The model under review builds one solid part; all positions refer to its coordinate system, in mm. Round coordinates to 2 decimals unless told otherwise and drop trailing zeros. Loops run counter-clockwise (first coordinate to the right, second up) from the corner with the lowest first, then second, coordinate; pieces in that order, holes last. Notation, with made-up numbers: M 82.25,17 L 123.25,17 A36 cw 123.25,51 Z; hole C -29.5,-22 d10. An arc over 180 degrees is marked long. Answer in a Markdown table with one row per item. Add a question column.
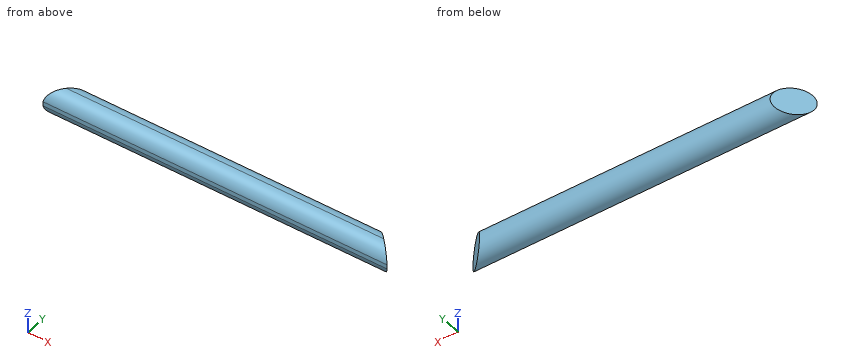
from build123d import *

# Parameters (mm, degrees)
SKETCH2_W               = 1600
SKETCH2_H               = 63.75
CUT_EXTRUDE2_DEPTH      = 1607.337546252
CUT_EXTRUDE2_DEPTH_BACK = 1607.337546252
CUT_EXTRUDE3_DEPTH      = 1607.337546252


with BuildPart() as part:
    # Sketch2 → Revolve1 (revolve)
    with BuildSketch(Plane(origin=(0, 0, 0), x_dir=(1, 0, 0), z_dir=(0, 1, 0))):
        with Locations((800, 31.875)):
            Rectangle(SKETCH2_W, SKETCH2_H)
    revolve(axis=Axis((1600, 0, -63.75), (-1, 0, 0)))

    # Sketch3 → Cut-Extrude2 (cut, two sides: drawn at the far end of the back side and taken through both)
    with BuildSketch(Plane.XY.offset(-CUT_EXTRUDE2_DEPTH_BACK)):
        Polygon((0, 63.75), (125, 63.75), (0, -63.75), align=None)
        Polygon((1600, 63.75), (1600, -63.75), (1475, 63.75), align=None)
    extrude(amount=CUT_EXTRUDE2_DEPTH + CUT_EXTRUDE2_DEPTH_BACK, mode=Mode.SUBTRACT)

    # Sketch5 → Cut-Extrude3 (cut, through all)
    with BuildSketch(Plane(origin=(0, 0, 0), x_dir=(0, 0, -1), z_dir=(1, 0, 0))):
        Polygon((63.75, -63.75), (0, -63.75), (0, -62.96232629), (127.5, -62.96232629), (127.5, -63.75), align=None)
    extrude(amount=CUT_EXTRUDE3_DEPTH, mode=Mode.SUBTRACT)


solid = part.part
1. Take a section at B-B, the plane x = 755.5. State the section outline as (y, z) points.
2. Take a section at C-C, the plane y = 49. State the section outline as (x, z) points, and give its area (3 significant figures).
3. Take a section at A-A, the plane z = -102. State the section outline as (x, y) points, and give its area (3 significant figures).
4. To check wall thickness, follow probe 1 along Z at (x, y) = (1393, 4); probe 2 along Z at (x, y) = (579.5, -1); probe 3 along Y at (x, z) = (494.5, -65). State the ranges of each line that lie inside material, in increasing order.
5. For pin 1 Ø6 at (y, z) = (-17.5, -22) entering from -X; pin 2 Ø2 at (x, y) = (384, -33) entering from +Z; pin 3 Ø1 at (x, y) = (670.5, 31) entering from -Z, all flat-tipped, find the tip position at first contact; note any pin that passes through.
Check sheet entries:
| question | item | result |
|---|---|---|
| 1 | outline | M -62.96,-73.74 A63.75 ccw long -62.96,-53.76 Z |
| 2 | outline | M 110.54,-104.53 L 1489.46,-104.53 L 1489.46,-22.97 L 110.54,-22.97 Z |
| 2 | area | 112,000 mm^2 |
| 3 | outline | M 12.5,-51 L 1587.5,-51 L 1487.5,51 L 112.5,51 Z |
| 3 | area | 150,000 mm^2 |
| 4 | probe 1 | z = -127.37 to -0.13 |
| 4 | probe 2 | z = -127.49 to -0.01 |
| 4 | probe 3 | y = -62.96 to 63.74 |
| 5 | pin 1 | stops at x = 42.4 |
| 5 | pin 2 | stops at z = -8.61 |
| 5 | pin 3 | stops at z = -119.73 |
